```python
from build123d import *

# Parameters (mm, degrees)
SKETCH_1_R          = 12
SKETCH_1_R_2        = 1.5
EXTRUDE_1_DEPTH     = 28
SKETCH_2_R          = 20
EXTRUDE_2_DEPTH     = 11
EXTRUDE_START       = -7.4
EXTRUDE_3_DEPTH     = 6.3
SKETCH_4_R          = 20
SKETCH_4_R_2        = 12
CUT_EXTRUDE_1_DEPTH = 39
CUT_EXTRUDE_START   = -1.5
SKETCH_5_R          = 12
CUT_EXTRUDE_2_DEPTH = 1.5
SKETCH_6_R          = 1.01
CUT_EXTRUDE_3_DEPTH = 1.5


with BuildPart() as part:
    # 草图1 → 凸台-拉伸1 (new body)
    with BuildSketch(Plane.XY):
        Circle(SKETCH_1_R)
        with Locations((-8, 0)):
            Circle(SKETCH_1_R_2, mode=Mode.SUBTRACT)
        with Locations(Location((8, 0, 0), (0, 0, 180))):
            Circle(SKETCH_1_R_2, mode=Mode.SUBTRACT)
        with Locations((0, 8)):
            Circle(SKETCH_1_R_2, mode=Mode.SUBTRACT)
        with Locations(Location((0, -8, 0), (0, 0, 180))):
            Circle(SKETCH_1_R_2, mode=Mode.SUBTRACT)
    extrude(amount=EXTRUDE_1_DEPTH)

    # 草图2 → 凸台-拉伸2 (add)
    with BuildSketch(Plane.XY.offset(28)):
        Circle(SKETCH_2_R)
    extrude(amount=-EXTRUDE_2_DEPTH)

    # 草图3 → 凸台-拉伸3 (add)
    with BuildSketch(Plane(origin=(0, 0, 0), x_dir=(-1, 0, 0), z_dir=(0, 0, -1)).offset(EXTRUDE_START)):
        with BuildLine():
            ThreePointArc((-4.178090404, -11.249158216), (-8.485281374, -8.485281374), (-11.249158216, -4.178090404))
            Line((-11.249158216, -4.178090404), (-25.39129384, -18.320226028))
            Line((-25.39129384, -18.320226028), (-18.320226028, -25.39129384))
            Line((-18.320226028, -25.39129384), (-4.178090404, -11.249158216))
        make_face()
    extrude(amount=-EXTRUDE_3_DEPTH)

    # 草图4 → 切除-拉伸1 (cut)
    with BuildSketch(Plane(origin=(0, 0, 17), x_dir=(-1, 0, 0), z_dir=(0, 0, -1))):
        Circle(SKETCH_4_R)
        with Locations(Location((0, 0, 0), (0, 0, 180))):
            Circle(SKETCH_4_R_2, mode=Mode.SUBTRACT)
    extrude(amount=-CUT_EXTRUDE_1_DEPTH, mode=Mode.SUBTRACT)

    # 草图5 → 切除-拉伸2 (cut)
    with BuildSketch(Plane.XY.offset(28).offset(CUT_EXTRUDE_START)):
        Circle(SKETCH_5_R)
    extrude(amount=CUT_EXTRUDE_2_DEPTH, mode=Mode.SUBTRACT)

    # 草图6 → 切除-拉伸3 (cut)
    with BuildSketch(Plane.XY.offset(26.5)):
        with Locations((5.5, 0)):
            Circle(SKETCH_6_R)
        with Locations((-2.75, -4.763139721)):
            Circle(SKETCH_6_R)
        with Locations((-2.75, 4.763139721)):
            Circle(SKETCH_6_R)
    extrude(amount=-CUT_EXTRUDE_3_DEPTH, mode=Mode.SUBTRACT)


solid = part.part
```
Input: part model. Units: mm. Frame: model coordinates. A direction names the side the tool comes from. Round coordinates to 2 decimals unless told otherwise and drop trailing zeros. Loops run counter-clockwise (first coordinate to the right, second up) from the corner with the lowest first, then second, coordinate; pieces in that order, holes last. Notation, with made-up numbers: (48, 45.25) - (87, 45.25) arc R26 cw to (87, 73.25) - close; hole circle Ø9 at (17, -2). An arc over 180 degrees is marked (long way). One line per item, written item: value. Start each with the question number.
(1) Section C-C, the plane x = 0. Return loops of the section in (y, z), plus the area to 3 significant figures.
(2) Draft query along Y for faces 5 (the flat face through (11.35, -18.42, 10.51)), 6 (the cylindrical face through (-2.969, 3.777, 25.76)), 7 (the flat face through (0, 0, 0)). Return one class per face: +Y half, -Y half, draft (parallel to the pull), parting line (faces both ways), or undercut.
(3) Contact query for flat-ended pins moving along their axis: P1, Ø1.5, axis at y = 0.5, z = 21, coming from the -X side; P2, Ø6, axis at y = -8.5, z = 22, coming from the -X side; P3, Ø1.2, axis at x = -2.75, y = -4.76, coming from the +Z side; P4, Ø17, axis at x = 18, y = -11, coming from the -Z side. Output: stop coordinate, or through.
(4) Section D-D, the plane z = 3.25. Return loops of the section in (x, y).
(5) Section B-B, the plane z = 8.75. Return loops of the section in (x, y).
(6) Section A-A, the plane y = 0. Return loops of the section in (x, z).
(7) Ray query, line 1 (Y direction, x = 0, z = 6.25); line 2 (X direction, y = -0.5, z = 10.25); line 3 (Y direction, x = -2.75, z = 26.1). Return the intervals inside material, ascending. Write a range as [from, to].
(8) Access query for faces 1 (the flat face through (-3, 5, 25)), 2 (the flat face through (0, 0, 26.5)), 3 (the cylindrical face through (-0.325, 6.536, 8.381)), 4 (the flat face through (15, -15, 13.7)). Directions: +Z, -Z, +X, -X, +Y, -Y. A direction counts if a zero-diameter tool reaches every point of the face in a straight line with its end or side. Return the directions, or none.
Results below:
1. outline: (-12, 0) - (-9.5, 0) - (-9.5, 17) - (-6.5, 17) - (-6.5, 0) - (6.5, 0) - (6.5, 17) - (9.5, 17) - (9.5, 0) - (12, 0) - (12, 26.5) - (-12, 26.5) - close
1. area: 534 mm^2
2. face 5: -Y half
2. face 6: undercut
2. face 7: draft
3. P1: x = -12
3. P2: x = -10.67
3. P3: z = 25
3. P4: z = 7.4
4. outline: circle Ø24 at (0, 0); hole circle Ø3 at (-8, 0); hole circle Ø3 at (0, -8); hole circle Ø3 at (0, 8); hole circle Ø3 at (8, 0)
5. outline: (4.18, -11.25) - (18.32, -25.39) - (25.39, -18.32) - (11.25, -4.18) arc R12 ccw (long way) to start; hole circle Ø3 at (-8, 0); hole circle Ø3 at (0, -8); hole circle Ø3 at (0, 8); hole circle Ø3 at (8, 0)
6. outline: (-12, 0) - (-9.5, 0) - (-9.5, 17) - (-6.5, 17) - (-6.5, 0) - (6.5, 0) - (6.5, 17) - (9.5, 17) - (9.5, 0) - (12, 0) - (12, 26.5) - (6.51, 26.5) - (6.51, 25) - (4.49, 25) - (4.49, 26.5) - (-12, 26.5) - close
7. line 1: [-12, -9.5], [-6.5, 6.5], [9.5, 12]
7. line 2: [-11.99, -9.41], [-6.59, 6.59], [9.41, 11.99]
7. line 3: [-11.68, -5.77], [-3.75, 3.75], [5.77, 11.68]
8. face 1: +Z
8. face 2: +Z, +X, -X, +Y, -Y
8. face 3: -Z
8. face 4: +Z, +X, -Y
